The listing builds one solid part. Answer for the finished solid, in the listing's coordinates (mm). Coordinates: 2 decimals unless noted, no trailing zeros. Order: outer loops, then holes, each group sorted by start corner. A loop starts at its lowest first (then second) coordinate and runs counter-clockwise, first axis right, second up. Notation, with made-up numbers: (-37.75, 38.25) -> (-8.75, 38.25) arc R36 cw to (-8.75, 75.25) -> close; hole circle Ø2 at (46.25, 85). An arc over 180 degrees is marked (long way). Answer in a Markdown table with one row per item.
Autodesk Inventor part; units mm, degrees
ref_plane "YZ Plane" through (0, 0, 0) normal (1, 0, 0) x (0, 1, 0)
ref_plane "XZ Plane" through (0, 0, 0) normal (0, 1, 0) x (-1, 0, 0)
ref_plane "XY Plane" through (0, 0, 0) normal (0, 0, 1) x (1, 0, 0)
sketch "Skizze1" plane through (0, 0, 0) normal (0, 1, 0) x (-1, 0, 0)
  point P0 (0, 0)
sketch "Skizze2" plane through (0, 0, 0) normal (0, 1, 0) x (-1, 0, 0)
  line L0 (15, 7.5) -> (-15, 7.5)
  line L1 (-15, 7.5) -> (-15, -7.5)
  line L2 (-15, -7.5) -> (15, -7.5)
  line L3 (15, -7.5) -> (15, 7.5)
  circle A0 centre (0, 0) radius 2.5
  dimension "d4" = 15
  dimension "d5" = 30
  dimension "d6" = 15
  dimension "d7" = 7.5
  dimension "d8" = 5
extrude "Extrusion1" add sketch "Skizze2" along normal blind 50
sketch "Skizze3" plane through (-15, 0, 7.5) normal (0, 0, 1) x (1, 0, 0)
  circle A0 centre (4, 10) radius 1.7
  circle A1 centre (4, 26) radius 1.7
  circle A2 centre (26, 10) radius 1.7
  circle A3 centre (26, 26) radius 1.7
  line L0 (30, 0) -> (30, 50)
  line L1 (0, 0) -> (0, 50)
  line L2 (0, 0) -> (30, 0)
  point P0 (15, 0)
  dimension "d11" = 22
  dimension "d12" = 3.4
  dimension "d13" = 3.4
  dimension "d14" = 3.4
  dimension "d15" = 3.4
  dimension "d16" = 4
  dimension "d17" = 16
  dimension "d18" = 4
  dimension "d19" = 16
  dimension "d20" = 4
  dimension "d21" = 22
  dimension "d22" = 10
extrude "Extrusion2" cut sketch "Skizze3" against normal blind 15
properties part number "Gegenstück Rotorachse"
(1) For a pull along X with two mould halves and no side action, classify faces 1 (the flat face through (15, 25, 0)), 2 (the flat face through (-15, 25, 0)), 3 (the cylindrical face through (-10.086, 27.433, 0.105)), 4 (the flat face through (4, 0, 0)) as released by +X, released by -X, zero draft, split by the parting line, or undercut.
Check values:
| item | result |
|---|---|
| face 1 | released by +X |
| face 2 | released by -X |
| face 3 | undercut |
| face 4 | zero draft |
(2) A cutting plane is placed at B-B, the plane z = 0. Determine the outline of the cut face in (x, y).
Check values:
| item | result |
|---|---|
| outline | (-15, 0) -> (-2.5, 0) -> (-2.5, 50) -> (-15, 50) -> close; (2.5, 0) -> (15, 0) -> (15, 50) -> (2.5, 50) -> close; hole circle Ø3.4 at (-11, 10); hole circle Ø3.4 at (-11, 26); hole circle Ø3.4 at (11, 10); hole circle Ø3.4 at (11, 26) |
(3) Find the intervals of material crossed by line 1 along Y through (x, z) = (11, 2); line 2 along Y through (x, z) = (-12.5, 3.25); line 3 along X through (y, z) = (7, -0.75), in increasing order. Write a range as from..to.
Check values:
| item | result |
|---|---|
| line 1 | 0..8.3, 11.7..24.3, 27.7..50 |
| line 2 | 0..9.2, 10.8..25.2, 26.8..50 |
| line 3 | -15..-2.38, 2.38..15 |
(4) A cutting plane is placed at A-A, the plane y = 10. Determine the outline of the cut face in (x, z), then the cut area to 3 significant figures.
Check values:
| item | result |
|---|---|
| outline | (-15, -7.5) -> (-12.7, -7.5) -> (-12.7, 7.5) -> (-15, 7.5) -> close; (-9.3, -7.5) -> (9.3, -7.5) -> (9.3, 7.5) -> (-9.3, 7.5) -> close; (12.7, -7.5) -> (15, -7.5) -> (15, 7.5) -> (12.7, 7.5) -> close; hole circle Ø5 at (0, 0) |
| area | 328 mm² |
(5) A cutting plane is placed at D-D, the plane z = 4. Determine the outline of the cut face in (x, y), then the cut area to 3 significant figures.
Check values:
| item | result |
|---|---|
| outline | (-15, 0) -> (15, 0) -> (15, 50) -> (-15, 50) -> close; hole circle Ø3.4 at (-11, 10); hole circle Ø3.4 at (-11, 26); hole circle Ø3.4 at (11, 10); hole circle Ø3.4 at (11, 26) |
| area | 1,460 mm² |
(6) A cutting plane is placed at C-C, the plane x = 1.5. Determine the outline of the cut face in (y, z).
Check values:
| item | result |
|---|---|
| outline | (0, -7.5) -> (50, -7.5) -> (50, -2) -> (0, -2) -> close; (0, 2) -> (50, 2) -> (50, 7.5) -> (0, 7.5) -> close |
(7) A flat-ended cylindrical pin translates along its axis: pin 1 (3 mm diameter, centred on x = 11, y = 26, fed in from -Z). Find the tip coordinate at first contact, or state that the pin passes through.
Check values:
| item | result |
|---|---|
| pin 1 | through |
